Design review of the part shown in the three views and the two pictorial views. Dimensions are in mm from the part's minimum x, y and z. A direction names the side the tool comes from. Round coordinates to 2 decimals unless told otherwise and drop trailing zeros. Order: outer loops, then holes, each group sorted by start corner. A loop starts at its lowest first (then second) coordinate and runs counter-clockwise, first axis right, second up. Notation, with made-up numbers: (-24.5, 25.5) - (7.5, 25.5) arc R16 cw to (7.5, 48.5) - close; hole circle Ø3 at (17.25, 54). An arc over 180 degrees is marked (long way). One line per item, written item: value.
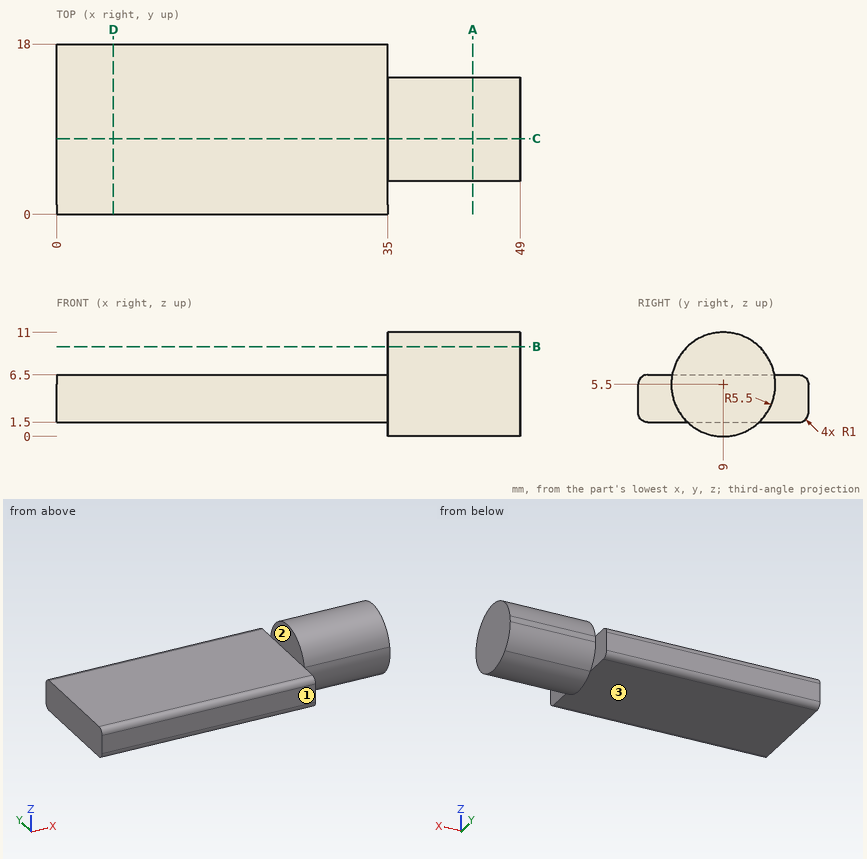
Item 1: Take a section at A-A (x = 44). Write out the cut boundary in (y, z).
Returned:
outline: circle Ø11 at (9, 5.5)
Item 2: Take a section at C-C (y = 8). Write out the cut boundary in (x, z).
Returned:
outline: (0, 1.5) - (35, 1.5) - (35, 0.09) - (49, 0.09) - (49, 10.91) - (35, 10.91) - (35, 6.5) - (0, 6.5) - close
Item 3: For P1, Ø3.5, axis at y = 7.5, z = 9.5, coming from the -X side; P2, Ø8, axis at x = 16, y = 12.5, coming from the -Z side; P3, Ø5, axis at x = 10.5, y = 14.5, coming from the +Z side, all flat-tipped, find the tip position at first contact; note any pin that passes through.
Returned:
P1: x = 35
P2: z = 1.5
P3: z = 6.5
Item 4: Take a section at B-B (z = 9.5). Write out the cut boundary in (x, y), plus the area to 3 significant figures.
Returned:
outline: (35, 5.23) - (49, 5.23) - (49, 12.77) - (35, 12.77) - close
area: 106 mm^2
Item 5: Wall thickness on line 1 (Y direction, x = 38.5, z = 5.75); line 2 (Z direction, x = 20.5, y = 10); line 3 (X direction, y = 16.5, z = 3.5): over which ranges is each line inside the solid? List them lowest first.
Returned:
line 1: 3.51 to 14.49
line 2: 1.5 to 6.5
line 3: 0 to 35
Item 6: Take a section at D-D (x = 6). Write out the cut boundary in (y, z), plus the area to 3 significant figures.
Returned:
outline: (0, 2.5) arc R1 ccw to (1, 1.5) - (17, 1.5) arc R1 ccw to (18, 2.5) - (18, 5.5) arc R1 ccw to (17, 6.5) - (1, 6.5) arc R1 ccw to (0, 5.5) - close
area: 89.1 mm^2
Item 7: Machinability: for the marked faces 1, 2 and 3, which of the approach directions +Z, -Z, +X, -X, +Y, -Y give a long, thin tool a straight path to every point of the face, cutting with its end or side? Answer none if there is none.
Returned:
face 1: +Z, -Z, +X, -X, -Y
face 2: +Z, -X, +Y, -Y
face 3: -Z, -X, +Y, -Y
